For this review, take the finished solid that the model builds, in its own axes (mm). Face numbers are marked on the shaded views. A direction names the side the tool comes from. Give positions to 0.01 mm unless a question says otherwise; leave off trailing zeros. Order: outer loops, then holes, each group sorted by start corner. A loop starts at its lowest first (then second) coordinate and runs counter-clockwise, first axis right, second up. Notation, with made-up numbers: (55.25, -17.5) - (91.25, -17.5) arc R23 ccw to (91.25, -1.5) - close; hole circle Ø5 at (58, 63). An arc over 180 degrees is marked (long way). Answer as a JSON object with one key per item and string values. Group by question number.
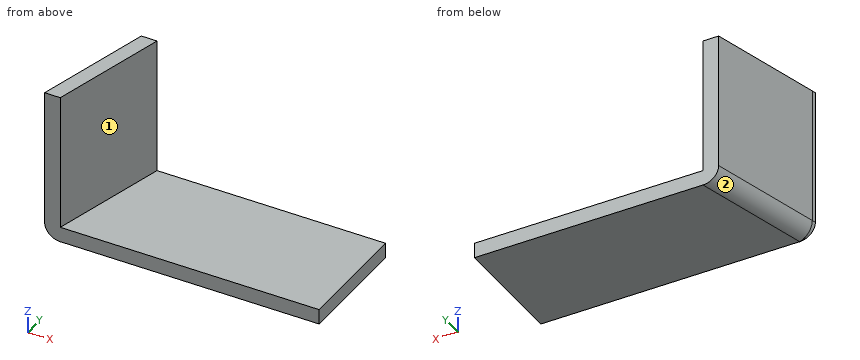
from build123d import *

# Parameters (mm, degrees)
BASE_FLANGE5_DEPTH       = 3.175
EDGE_FLANGE4_START       = -37.332955736
EDGE_FLANGE4_DEPTH       = 25.4
BOSS_EXTRUDE3_DEPTH      = 28.575
BOSS_EXTRUDE3_DEPTH_BACK = 5.08
CUT_EXTRUDE4_DEPTH       = 34.925
CUT_EXTRUDE4_DEPTH_BACK  = 5.588
CUT_EXTRUDE7_DEPTH       = 33.274
CUT_EXTRUDE7_DEPTH_BACK  = 9.779


# Read off the part's stored shape, not the designer's step: Edge-Flange4
# Sheet-metal steps are written as plain solids
with BuildPart() as part:
    # Sketch13 → Base-Flange5 (new body)
    with BuildSketch(Plane.XY):
        Polygon((-47.732145582, 0), (0, 0), (0, -24.593455331), (-54.08210266, -24.593455331), align=None)
    extrude(amount=-BASE_FLANGE5_DEPTH)

    # Edge-Flange4 outline → Edge-Flange4 (add)
    with BuildSketch(Plane(origin=(0, 0, 0), x_dir=(0.9682462728649326, -0.24999831016062188, 0), z_dir=(0.24999831016062188, 0.9682462728649326, 0)).offset(EDGE_FLANGE4_START)):
        with BuildLine():
            Line((-46.216472056, -28.575), (-46.216472056, 3.175))
            ThreePointArc((-46.216472056, 3.175), (-48.461536086, 2.24506403), (-49.391472056, 0))
            Line((-49.391472056, 0), (-49.391472056, -28.575))
            Line((-49.391472056, -28.575), (-46.216472056, -28.575))
        make_face()
    extrude(amount=EDGE_FLANGE4_DEPTH)

    # Sketch50 → Boss-Extrude3 (add, two sides: drawn at the far end of the back side and taken through both)
    with BuildSketch(Plane.XY.offset(-BOSS_EXTRUDE3_DEPTH_BACK)):
        Polygon((-54.08210266, -24.593455331), (-57.156284576, -23.799710696), (-57.361227082, -24.593455331), align=None)
    extrude(amount=BOSS_EXTRUDE3_DEPTH + BOSS_EXTRUDE3_DEPTH_BACK)

    # Sketch51 → Cut-Extrude4 (cut, two sides: drawn at the far end of the back side and taken through both)
    with BuildSketch(Plane.XY.offset(-CUT_EXTRUDE4_DEPTH_BACK)):
        Polygon((-47.732145582, 0), (-51.011270004, 0), (-50.806327498, 0.793744635), align=None)
    extrude(amount=CUT_EXTRUDE4_DEPTH + CUT_EXTRUDE4_DEPTH_BACK, mode=Mode.SUBTRACT)

    # Sketch56 → Cut-Extrude7 (cut, two sides: drawn at the far end of the back side and taken through both)
    with BuildSketch(Plane(origin=(-9.298174, -36.122285036, -0.026223985), x_dir=(0.9684252131455058, -0.24928299754212324, 0.0032547934643607206), z_dir=(0.24928204027092418, 0.9684306738770053, 0.0007030593821182495)).offset(-CUT_EXTRUDE7_DEPTH_BACK)):
        with BuildLine():
            Line((-49.435258201, 4.892901472), (-46.260275882, 4.90323379))
            Line((-46.260275882, 4.90323379), (-46.235347228, 3.016163107))
            ThreePointArc((-46.235347228, 3.016163107), (-48.4905831, 2.0739806), (-49.418723851, -0.187070364))
            Line((-49.418723851, -0.187070364), (-50.079202572, -0.187070364))
            Line((-50.079202572, -0.187070364), (-50.079202572, 4.892901472))
            Line((-50.079202572, 4.892901472), (-49.435258201, 4.892901472))
        make_face()
    extrude(amount=CUT_EXTRUDE7_DEPTH + CUT_EXTRUDE7_DEPTH_BACK, mode=Mode.SUBTRACT)


solid = part.part
1) For pin 1 (4 mm diameter, centred on x = -30, y = -10, fed in from +Z); pin 2 (10 mm diameter, centred on y = -7, z = 17, fed in from +X); pin 3 (1 mm diameter, centred on x = -27.5, y = -21.5, fed in from -Z) (3 decimals), all flat-tipped, find the tip position at first contact; note any pin that passes through.
2) For the marked faces 1 and 2, list the 3-axis set-ups (+Z, -Z, +X, -X, +Y, -Y) from which the entire face can be reached by the end or side of a thin tool; tool diameter is ignored.
3) Consider section A-A (z = 15). Give the boundary of the cut face in (x, y).
4) Consider section B-B (x = -31). Give the boundary of the cut face in (y, z) (3 decimals), plus the area to 3 significant figures.
5) For line 1 (Z direction, x = -28, y = -2) (3 decimals); line 2 (X direction, y = -23, z = 12); line 3 (X direction, y = -8.75, z = 21.5), list the stretches that pass through material, from the lowest coordinate up.
Result set:
{
 "1": {"pin 1": "stops at z = 0", "pin 2": "stops at x = -48.25", "pin 3": "stops at z = -3.175"},
 "2": {"face 1": "+Z, +X, -Y", "face 2": "-Z, -X, +Y"},
 "3": {"outline": "(-57.36, -24.59) - (-54.08, -24.59) - (-47.73, 0) - (-51.01, 0) - close"},
 "4": {"outline": "(-24.593, -3.175) - (0, -3.175) - (0, 0) - (-24.593, 0) - close", "area": "78.1 mm2"},
 "5": {"line 1": "z = -3.175 to 0", "line 2": "x = -56.95 to -53.67", "line 3": "x = -53.27 to -49.99"}
}
